Check sheet for the modelled part. Datum: model origin and axes. Units: mm. Face numbers are marked on the shaded views. A direction names the side the tool comes from. Coordinates: 2 decimals unless noted, no trailing zeros. Loops run counter-clockwise (first coordinate to the right, second up) from the corner with the lowest first, then second, coordinate; pieces in that order, holes last.
```python
from build123d import *

# Parameters (mm, degrees)
BOSS_EXTRUDE1_DEPTH = 3.175
CUT_EXTRUDE1_DEPTH  = 46.155334956


with BuildPart() as part:
    # Sketch2 → Boss-Extrude1 (new body)
    with BuildSketch(Plane(origin=(0, 0, 0), x_dir=(1, 0, 0), z_dir=(0, 1, 0))):
        with BuildLine():
            Line((-5.582827527, 34.123976372), (-4.37531266, 30.407627744))
            ThreePointArc((-4.37531266, 30.407627744), (-6.673596197, 26.127217151), (-11.454717255, 25.264139232))
            Line((-11.454717255, 25.264139232), (-14.61603222, 27.560968998))
            ThreePointArc((-14.61603222, 27.560968998), (-21.427113101, 23.90389108), (-18.066409385, 16.9418))
            Line((-18.066409385, 16.9418), (-14.15880919, 16.9418))
            ThreePointArc((-14.15880919, 16.9418), (-10.798105475, 13.433282849), (-11.454717255, 8.619460768))
            Line((-11.454717255, 8.619460768), (-14.61603222, 6.322631002))
            ThreePointArc((-14.61603222, 6.322631002), (-13.242684177, -1.28519108), (-5.582827527, -0.240376372))
            Line((-5.582827527, -0.240376372), (-4.37531266, 3.475972256))
            ThreePointArc((-4.37531266, 3.475972256), (0, 5.588), (4.37531266, 3.475972256))
            Line((4.37531266, 3.475972256), (5.582827527, -0.240376372))
            ThreePointArc((5.582827527, -0.240376372), (13.242684177, -1.28519108), (14.61603222, 6.322631002))
            Line((14.61603222, 6.322631002), (11.454717255, 8.619460768))
            ThreePointArc((11.454717255, 8.619460768), (10.798105475, 13.433282849), (14.15880919, 16.9418))
            Line((14.15880919, 16.9418), (18.066409385, 16.9418))
            ThreePointArc((18.066409385, 16.9418), (21.427113101, 23.90389108), (14.61603222, 27.560968998))
            Line((14.61603222, 27.560968998), (11.454717255, 25.264139232))
            ThreePointArc((11.454717255, 25.264139232), (6.673596197, 26.127217151), (4.37531266, 30.407627744))
            Line((4.37531266, 30.407627744), (5.582827527, 34.123976372))
            ThreePointArc((5.582827527, 34.123976372), (0, 39.4716), (-5.582827527, 34.123976372))
        make_face()
    extrude(amount=BOSS_EXTRUDE1_DEPTH)

    # Sketch3 → Cut-Extrude1 (cut, through all)
    with BuildSketch(Plane(origin=(0, 3.175, 0), x_dir=(1, 0, 0), z_dir=(0, 1, 0))):
        with BuildLine():
            Line((-0.933255592, 15.381358575), (0.933255592, 15.381358575))
            ThreePointArc((0.933255592, 15.381358575), (0, 16.905358575), (-0.933255592, 15.381358575))
        make_face()
    extrude(amount=-CUT_EXTRUDE1_DEPTH, mode=Mode.SUBTRACT)


solid = part.part
```
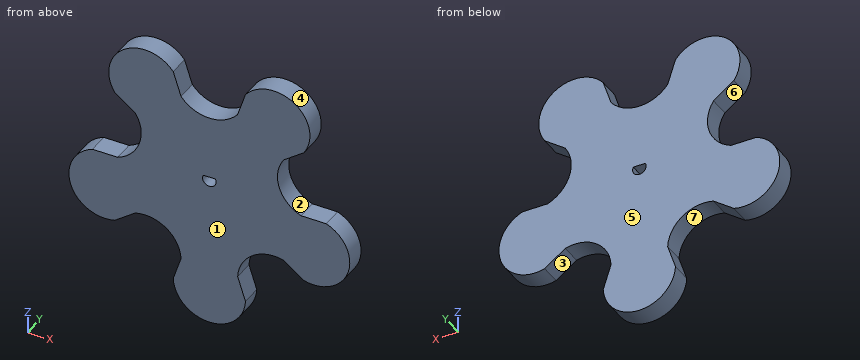
1) Set-up check for the marked faces 5, 6 and 7: record each of +Z, -Z, +X, -X, +Y, -Y from which the full face is reachable in a straight line by a thin tool's end or side.
Answer sheet:
face 5: +Z, -Z, +X, -X, +Y
face 6: -X, +Y, -Y
face 7: +Y, -Y
2) Mould release check, pull along X, two halves, no side actions. Record for the marked faces 1, 2, 3 and 4: +X half, -X half, draft (parallel to the pull), parting line (faces both ways), or undercut.
Answer sheet:
face 1: draft
face 2: +X half
face 3: undercut
face 4: undercut
3) Depth check by flat-ended pin: pin 1 (1.9 mm diameter, centred on x = 0, z = -15.86, fed in from -Y); pin 2 (1.6 mm diameter, centred on x = -16.5, y = 1, fed in from +Z); pin 3 (0.6 mm diameter, centred on x = 0.5, y = 2.5, fed in from -Z); pin 4 (1 mm diameter, centred on x = 1.5, y = 2.5, fed in from -Z). Enter the tip coordinate at first touch or a pass-through.
Answer sheet:
pin 1: stops at y = 0
pin 2: stops at z = -16.94
pin 3: stops at z = -39.47
pin 4: stops at z = -39.38
4) Scan lines: line 1 (Z direction, x = 11, y = 2.9); line 2 (Z direction, x = -0.5, y = 1.95); line 3 (X direction, y = 1.55, z = -11.5). Record each from-to range of solid material in increasing order.
Answer sheet:
line 1: z = -25.16 to -13.96, -9.45 to 2.25
line 2: z = -39.45 to -16.78, -15.38 to -5.57
line 3: x = -10.53 to 10.53
5) Section check C-C on z = -16. Enter the section's corners in (x, y) (3 decimals), plus the area to 3 significant figures.
Answer sheet:
outline: (-12.536, 0) - (-1.038, 0) - (-1.038, 3.175) - (-12.536, 3.175) - close; (1.038, 0) - (12.536, 0) - (12.536, 3.175) - (1.038, 3.175) - close
area: 73.0 mm2
6) Section check A-A on x = 0. Enter the section's corners in (y, z) (3 decimals).
Answer sheet:
outline: (0, -39.472) - (3.175, -39.472) - (3.175, -16.905) - (0, -16.905) - close; (0, -15.381) - (3.175, -15.381) - (3.175, -5.588) - (0, -5.588) - close
7) Section check B-B on y = 2.6. Enter the section's corners in (x, z).
Answer sheet:
outline: (-18.07, -16.94) arc R5.59 ccw to (-14.62, -27.56) - (-11.45, -25.26) arc R5.59 cw to (-4.38, -30.41) - (-5.58, -34.12) arc R5.59 ccw to (5.58, -34.12) - (4.38, -30.41) arc R5.59 cw to (11.45, -25.26) - (14.62, -27.56) arc R5.59 ccw to (18.07, -16.94) - (14.16, -16.94) arc R5.59 cw to (11.45, -8.62) - (14.62, -6.32) arc R5.59 ccw to (5.58, 0.24) - (4.38, -3.48) arc R5.59 cw to (-4.38, -3.48) - (-5.58, 0.24) arc R5.59 ccw to (-14.62, -6.32) - (-11.45, -8.62) arc R5.59 cw to (-14.16, -16.94) - close; hole (-0.93, -15.38) arc R1.05 ccw (long way) to (0.93, -15.38) - close
8) Section check D-D on z = -35. Enter the section's corners in (x, y) (3 decimals).
Answer sheet:
outline: (-5.475, 0) - (5.475, 0) - (5.475, 3.175) - (-5.475, 3.175) - close
